Build history of the part. All positions in model axes, mm. Round coordinates to 2 decimals unless told otherwise and drop trailing zeros. Loops run counter-clockwise (first coordinate to the right, second up) from the corner with the lowest first, then second, coordinate; pieces in that order, holes last. Notation, with made-up numbers: (-24.5, -39) - (33.5, -39) arc R14 cw to (33.5, -14) - close; hole circle Ø7 at (61.25, 48). An arc over 180 degrees is marked (long way). Use one line per item in the form item = value. Start each with the question number.
Q1. Drill centre lines: line 1 (Z direction, x = -8.5, y = -9.75); line 2 (Z direction, x = -7, y = 6.75); line 3 (Y direction, x = -1.75, z = 6.5). Where is each one in solid material? Low to high.
Q2. Saw through at A-A (x = -3.5). Give the cut face in (y, z), then the cut area to 3 significant figures.
Q3. Saw through at D-D (z = -6). Give the cut face in (x, y), then the cut area to 3 significant figures.
Q4. Saw through at B-B (y = 3.25). Give the cut face in (x, z), then the cut area to 3 significant figures.
Q5. Saw through at C-C (z = -15). Give the cut face in (x, y), then the cut area to 3 significant figures.
Q6. Pin check, flat tips, straight feed: pin 1 (2 mm diameter, centred on x = 2, y = -3.5, fed in from +Z); pin 2 (6 mm diameter, centred on x = -2.5, z = -8.5, fed in from -Y); pin 3 (5 mm diameter, centred on x = 8, y = -6, fed in from +Z). Stop position of each tip, or through.
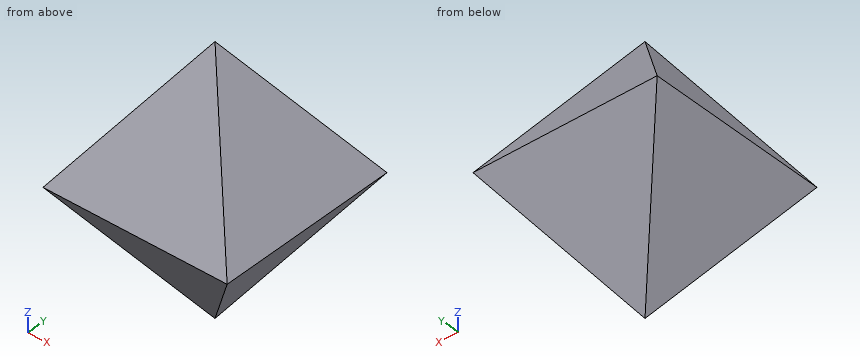
```python
from build123d import *

# Parameters (mm, degrees)
F0_W      = 25.4
F0_H      = 25.4
F1_DEPTH  = 25.4
F1_TAPER  = 35
F1_FACE_W = 25.4
F1_FACE_H = 25.4


# Not quite as in the source:
# - an extrude whose draft closes it to a point is written as a loft to that point


with BuildPart() as f1:
    # F0 (on Top) → F1 (new body)
    with BuildSketch(Plane.XY):
        Rectangle(F0_W, F0_H)
    extrude(amount=F1_DEPTH, taper=F1_TAPER)

    # F1_face (on face) → F2 section 0
    with BuildSketch(Plane(origin=(0, 0, 0), x_dir=(1, 0, 0), z_dir=(0, 0, -1)), mode=Mode.PRIVATE) as f2_s0:
        Rectangle(F1_FACE_W, F1_FACE_H)
    loft([f2_s0.sketch, Vertex(0, 0, -18.1374796856)], ruled=True)


solid = f1.part
```
Report:
q1.line_1 = -4.21 to 4.21
q1.line_2 = -8.14 to 8.14
q1.line_3 = -8.15 to 8.15
q2.outline = (-12.7, 0) - (-3.5, -13.14) - (3.5, -13.14) - (12.7, 0) - (3.5, 13.14) - (-3.5, 13.14) - close
q2.area = 426 mm²
q3.outline = (-8.5, -8.5) - (8.5, -8.5) - (8.5, 8.5) - (-8.5, 8.5) - close
q3.area = 289 mm²
q4.outline = (-12.7, 0) - (-3.25, -13.5) - (3.25, -13.5) - (12.7, 0) - (3.25, 13.5) - (-3.25, 13.5) - close
q4.area = 431 mm²
q5.outline = (-2.2, -2.2) - (2.2, -2.2) - (2.2, 2.2) - (-2.2, 2.2) - close
q5.area = 19.3 mm²
q6.pin_1 = 14.57
q6.pin_2 = -8.85
q6.pin_3 = 10.22
